Can you work these out from the model? Positions are in its coordinate system, mm. A direction names the side the tool comes from. Coordinates: 2 decimals unless noted, no trailing zeros. Loops run counter-clockwise (first coordinate to the right, second up) from the corner with the lowest first, then second, coordinate; pieces in that order, holes last. Notation, with made-up numbers: (-26.5, 85) -> (22.5, 85) arc R33 cw to (22.5, 120) -> close; hole circle Ø5 at (49, 29.25). An arc over 180 degrees is marked (long way). Put each result on its own line as item: value. Start each with the question number.
Item 1: If we section it at C-C on y = 4: Please give me the cut outline in (x, z).
Item 2: We'd pull the mould along Y, two halves only. Please class faces 3 (the flat face through (9, 0, -3)), 4 (the flat face through (13, 0, 0)): pulls with the +Y half, pulls with the -Y half, needs draft (parallel to the pull), parting line crosses it, or undercut.
Item 3: Will these pins go through, and if not, where does the flat tip stop? P1, Ø4, axis at x = 11, y = 3, coming from the -Z side; P2, Ø1.5, axis at x = 7.5, y = 2, coming from the +Z side; P3, Ø1.5, axis at y = -0.5, z = 0.5, coming from the -X side.
Item 4: Please list where these lines run through material, in increasing order: L1, parallel to Y at x = 8.5, z = 0; L2, parallel to Y at x = 7, z = -3.5; L3, parallel to X at y = 3, z = -4. Write a range as from..to.
Item 5: For faces 1 (the flat face through (8, -1, 3)), 2 (the cylindrical face through (11.03, 0.07, -1.7)), which set-ups out of +Z, -Z, +X, -X, +Y, -Y let a thin tool reach every point of the face, with its end or its side?
Item 6: If we section it at B-B on x = 12.5: Please give me the cut outline in (y, z), plus the area to 3 significant figures.
Item 7: If we section it at D-D on z = -3.2: Please give me the cut outline in (x, y), plus the area to 3 significant figures.
Item 8: If we section it at A-A on z = 0: Please give me the cut outline in (x, y).
```python
from build123d import *

# Parameters (mm, degrees)
BASPROSKE_W         = 8
BASPROSKE_H         = 4.8
TOOTHCUT_DEPTH      = 11.491901639
TEETHCUTS_COUNT     = 10
BORSKE_R            = 0.4
BORE_DEPTH          = 18.0000508
SKETCH1_R           = 6
BOSS_EXTRUDE1_DEPTH = 5
CUT_EXTRUDE1_DEPTH  = 5
SKETCH4_R           = 1.5
CUT_EXTRUDE2_DEPTH  = 7
SKETCH8_R           = 1.5
CUT_EXTRUDE8_DEPTH  = 4


with BuildPart() as part:
    # BasProSke → Base-Revolve (revolve)
    with BuildSketch(Plane(origin=(0, 0, 0), x_dir=(1, 0, 0), z_dir=(0, 1, 0)), mode=Mode.PRIVATE) as base_revolve_sk:
        with Locations((4, 2.4)):
            Rectangle(BASPROSKE_W, BASPROSKE_H)
    revolve(base_revolve_sk.sketch.rotate(Axis((-10, 0, 0), (1, 0, 0)), 180), axis=Axis((-10, 0, 0), (1, 0, 0)))

    # TooCutSke → ToothCut (cut, through all)
    with BuildSketch(Plane(origin=(0, 0, 0), x_dir=(0, 0, -1), z_dir=(1, 0, 0))):
        with BuildLine():
            ThreePointArc((0.473726058, 2.961348446), (0, 2.999), (-0.473726058, 2.961348446))
            ThreePointArc((-0.473726058, 2.961348446), (-0.678470427, 3.942691912), (-1.42693485, 4.6095924))
            ThreePointArc((-1.42693485, 4.6095924), (0, 4.8254), (1.42693485, 4.6095924))
            ThreePointArc((1.42693485, 4.6095924), (0.678470427, 3.942691912), (0.473726058, 2.961348446))
        make_face()
    toothcut = extrude(amount=TOOTHCUT_DEPTH, mode=Mode.SUBTRACT)

    # TeethCuts: ToothCut ×10 about axis
    teethcuts_axis = Axis((0, 0, 0), (1, 0, 0))
    for i in range(1, TEETHCUTS_COUNT):
        add(toothcut.rotate(teethcuts_axis, i * 360 / TEETHCUTS_COUNT), mode=Mode.SUBTRACT)

    # BorSke → Bore (cut, symmetric)
    with BuildSketch(Plane(origin=(0, 0, 0), x_dir=(0, 0, -1), z_dir=(1, 0, 0))):
        with Locations(Location((0, 0, 0), (0, 0, 180))):
            Circle(BORSKE_R)
    extrude(amount=BORE_DEPTH, both=True, mode=Mode.SUBTRACT)

    # Sketch1 → Boss-Extrude1 (add)
    with BuildSketch(Plane(origin=(8, 0, 0), x_dir=(0, 0, -1), z_dir=(1, 0, 0))):
        Circle(SKETCH1_R)
    extrude(amount=BOSS_EXTRUDE1_DEPTH)

    # Sketch2 → Cut-Extrude1 (cut)
    with BuildSketch(Plane.ZY):
        with BuildLine():
            ThreePointArc((-2.96279914, 0.464566741), (-3.940487364, 0.57700657), (-4.799040651, 0.09596267))
            ThreePointArc((-4.799040651, 0.09596267), (-4.8, 0), (-4.799040651, -0.09596267))
            ThreePointArc((-4.799040651, -0.09596267), (-3.940487364, -0.57700657), (-2.96279914, -0.464566741))
            ThreePointArc((-2.96279914, -0.464566741), (-2.852218492, -0.926741966), (-2.670020334, -1.365647251))
            ThreePointArc((-2.670020334, -1.365647251), (-3.527077196, -1.849352238), (-3.938910885, -2.743169889))
            ThreePointArc((-3.938910885, -2.743169889), (-3.883281573, -2.821369211), (-3.826100001, -2.898440751))
            ThreePointArc((-3.826100001, -2.898440751), (-2.848765291, -2.782968481), (-2.123889376, -2.117332029))
            ThreePointArc((-2.123889376, -2.117332029), (-1.762767972, -2.426241966), (-1.357384512, -2.67423041))
            ThreePointArc((-1.357384512, -2.67423041), (-1.76644342, -3.569321349), (-1.574251041, -4.534504787))
            ThreePointArc((-1.574251041, -4.534504787), (-1.483281573, -4.565071278), (-1.391719195, -4.593812979))
            ThreePointArc((-1.391719195, -4.593812979), (-0.668911703, -3.925931021), (-0.473726058, -2.961348446))
            ThreePointArc((-0.473726058, -2.961348446), (0, -2.999), (0.473726058, -2.961348446))
            ThreePointArc((0.473726058, -2.961348446), (0.668911703, -3.925931021), (1.391719195, -4.593812979))
            ThreePointArc((1.391719195, -4.593812979), (1.483281573, -4.565071278), (1.574251041, -4.534504787))
            ThreePointArc((1.574251041, -4.534504787), (1.76644342, -3.569321349), (1.357384512, -2.67423041))
            ThreePointArc((1.357384512, -2.67423041), (1.762767972, -2.426241966), (2.123889376, -2.117332029))
            ThreePointArc((2.123889376, -2.117332029), (2.848765291, -2.782968481), (3.826100001, -2.898440751))
            ThreePointArc((3.826100001, -2.898440751), (3.883281573, -2.821369211), (3.938910885, -2.743169889))
            ThreePointArc((3.938910885, -2.743169889), (3.527077196, -1.849352238), (2.670020334, -1.365647251))
            ThreePointArc((2.670020334, -1.365647251), (2.852218492, -0.926741966), (2.96279914, -0.464566741))
            ThreePointArc((2.96279914, -0.464566741), (3.940487364, -0.57700657), (4.799040651, -0.09596267))
            ThreePointArc((4.799040651, -0.09596267), (4.8, 0), (4.799040651, 0.09596267))
            ThreePointArc((4.799040651, 0.09596267), (3.940487364, 0.57700657), (2.96279914, 0.464566741))
            ThreePointArc((2.96279914, 0.464566741), (2.852218492, 0.926741966), (2.670020334, 1.365647251))
            ThreePointArc((2.670020334, 1.365647251), (3.527077196, 1.849352238), (3.938910885, 2.743169889))
            ThreePointArc((3.938910885, 2.743169889), (3.883281573, 2.821369211), (3.826100001, 2.898440751))
            ThreePointArc((3.826100001, 2.898440751), (2.848765291, 2.782968481), (2.123889376, 2.117332029))
            ThreePointArc((2.123889376, 2.117332029), (1.762767972, 2.426241966), (1.357384512, 2.67423041))
            ThreePointArc((1.357384512, 2.67423041), (1.76644342, 3.569321349), (1.574251041, 4.534504787))
            ThreePointArc((1.574251041, 4.534504787), (1.483281573, 4.565071278), (1.391719195, 4.593812979))
            ThreePointArc((1.391719195, 4.593812979), (0.668911703, 3.925931021), (0.473726058, 2.961348446))
            ThreePointArc((0.473726058, 2.961348446), (0, 2.999), (-0.473726058, 2.961348446))
            ThreePointArc((-0.473726058, 2.961348446), (-0.668911703, 3.925931021), (-1.391719195, 4.593812979))
            ThreePointArc((-1.391719195, 4.593812979), (-1.483281573, 4.565071278), (-1.574251041, 4.534504787))
            ThreePointArc((-1.574251041, 4.534504787), (-1.76644342, 3.569321349), (-1.357384512, 2.67423041))
            ThreePointArc((-1.357384512, 2.67423041), (-1.762767972, 2.426241966), (-2.123889376, 2.117332029))
            ThreePointArc((-2.123889376, 2.117332029), (-2.848765291, 2.782968481), (-3.826100001, 2.898440751))
            ThreePointArc((-3.826100001, 2.898440751), (-3.883281573, 2.821369211), (-3.938910885, 2.743169889))
            ThreePointArc((-3.938910885, 2.743169889), (-3.527077196, 1.849352238), (-2.670020334, 1.365647251))
            ThreePointArc((-2.670020334, 1.365647251), (-2.852218492, 0.926741966), (-2.96279914, 0.464566741))
        make_face()
    extrude(amount=-CUT_EXTRUDE1_DEPTH, mode=Mode.SUBTRACT)

    # Sketch4 → Cut-Extrude2 (cut)
    with BuildSketch(Plane.ZY.offset(-5)):
        Circle(SKETCH4_R)
    extrude(amount=-CUT_EXTRUDE2_DEPTH, mode=Mode.SUBTRACT)

    # Sketch8 → Cut-Extrude8 (cut)
    with BuildSketch(Plane(origin=(13, 0, 0), x_dir=(0, 0, -1), z_dir=(1, 0, 0))):
        with Locations((3.2, 0)):
            Circle(SKETCH8_R)
    extrude(amount=-CUT_EXTRUDE8_DEPTH, mode=Mode.SUBTRACT)


solid = part.part
```
Solutions:
1. outline: (5, -1.76) -> (8, -1.76) -> (8, -4.47) -> (13, -4.47) -> (13, 4.47) -> (8, 4.47) -> (8, 1.76) -> (5, 1.76) -> (5, 0.71) -> (8, 0.71) -> (8, -0.71) -> (5, -0.71) -> close
2. face 3: undercut
2. face 4: needs draft
3. P1: z = -5.92
3. P2: z = 5.82
3. P3: x = 12
4. L1: -6..-1.5, 1.5..6
4. L2: -2.93..-1.82, -0.6..0.6, 1.82..2.93
4. L3: 8..13
5. face 1: -X
5. face 2: +X
6. outline: circle Ø12 at (0, 0); hole circle Ø3 at (0, -3.2)
6. area: 106 mm^2
7. outline: (5, -2.9) -> (8, -2.9) -> (8, -5.08) -> (13, -5.08) -> (13, -1.5) -> (9, -1.5) -> (9, 1.5) -> (13, 1.5) -> (13, 5.08) -> (8, 5.08) -> (8, 2.9) -> (5, 2.9) -> (5, 1.58) -> (8, 1.58) -> (8, 0.55) -> (5, 0.55) -> (5, -0.55) -> (8, -0.55) -> (8, -1.58) -> (5, -1.58) -> close
7. area: 50.0 mm^2
8. outline: (5, -3) -> (8, -3) -> (8, -6) -> (13, -6) -> (13, 6) -> (8, 6) -> (8, 3) -> (5, 3) -> (5, 1.5) -> (12, 1.5) -> (12, -1.5) -> (5, -1.5) -> close
